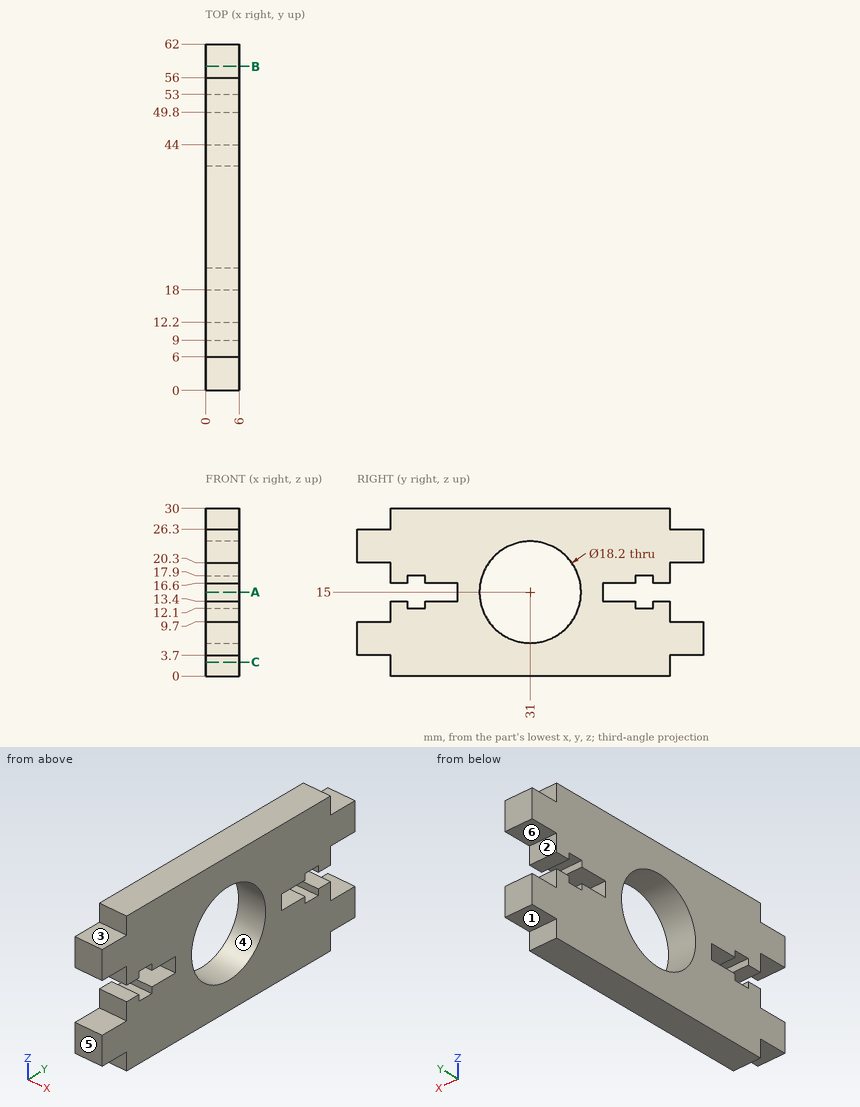
Geometry check sheet. Reference: drawing and pictorial views, mm from the part's lowest x, y, z. A direction names the side the tool comes from. Round coordinates to 2 decimals unless told otherwise and drop trailing zeros. Loops run counter-clockwise (first coordinate to the right, second up) from the corner with the lowest first, then second, coordinate; pieces in that order, holes last. Notation, with made-up numbers: (49.5, 49.5) -> (89.5, 49.5) arc R16 ccw to (89.5, 58.5) -> close; hole circle Ø9 at (71.25, 18.25). An arc over 180 degrees is marked (long way). Use a Markdown table: item, result.
(1) Set-up check for the marked faces 1, 2 and 3: record each of +Z, -Z, +X, -X, +Y, -Y from which the full face is reachable in a straight line by a thin tool's end or side.
Calculated:
| item | result |
|---|---|
| face 1 | -Z, +X, -X, +Y |
| face 2 | +X, -X, +Y |
| face 3 | +Z, +X, -X, -Y |
(2) Go/stop test with flat-tipped pins: P1, Ø1, axis at x = 4, z = 17.5, coming from the -Y side; P2, Ø1.4, axis at x = 1.5, z = 17.5, coming from the +Y side; P3, Ø3, axis at x = 2, y = 3.5, coming from the -Z side. Record where each tip stops, or that it passes through.
Calculated:
| item | result |
|---|---|
| P1 | y = 6 |
| P2 | y = 56 |
| P3 | z = 3.7 |
(3) Sectioned sample at B-B (y = 58). Enter the section's corners in (x, z), then the cut area to 3 significant figures.
Calculated:
| item | result |
|---|---|
| outline | (0, 3.7) -> (6, 3.7) -> (6, 9.7) -> (0, 9.7) -> close; (0, 20.3) -> (6, 20.3) -> (6, 26.3) -> (0, 26.3) -> close |
| area | 72.0 mm² |
(4) Sectioned sample at A-A (z = 15). Enter the section's corners in (x, y).
Calculated:
| item | result |
|---|---|
| outline | (0, 18) -> (6, 18) -> (6, 21.9) -> (0, 21.9) -> close; (0, 40.1) -> (6, 40.1) -> (6, 44) -> (0, 44) -> close |
(5) Scan lines: probe 1 along Y at (x, z) = (3.6, 14.75); probe 2 along Y at (x, z) = (5.4, 20.5); probe 3 along Z at (x, y) = (2.45, 45). Record each from-to range of solid material in increasing order.
Calculated:
| item | result |
|---|---|
| probe 1 | 18 to 21.9, 40.1 to 44 |
| probe 2 | 0 to 23.75, 38.25 to 62 |
| probe 3 | 0 to 13.4, 16.6 to 30 |
(6) Mould release check, pull along Y, two halves, no side actions. Record for the marked faces 4, 5 and 6: released by +Y, released by -Y, zero draft, split by the parting line, or undercut.
Calculated:
| item | result |
|---|---|
| face 4 | undercut |
| face 5 | released by -Y |
| face 6 | zero draft |
(7) Sectioned sample at C-C (z = 2.5). Enter the section's corners in (x, y), then the cut area to 3 significant figures.
Calculated:
| item | result |
|---|---|
| outline | (0, 6) -> (6, 6) -> (6, 56) -> (0, 56) -> close |
| area | 300 mm² |
